from build123d import *

# Parameters (mm, degrees)
SKETCH1_W           = 72
SKETCH1_H           = 39
BOSS_EXTRUDE1_DEPTH = 1.5
SKETCH2_R           = 10
BOSS_EXTRUDE2_DEPTH = 16.8
SKETCH3_R           = 1.6
CUT_EXTRUDE1_DEPTH  = 16.8
SKETCH4_R           = 1.6
CUT_EXTRUDE2_DEPTH  = 16.8
FILLET1_R           = 0.2


with BuildPart() as part:
    # Sketch1 → Boss-Extrude1 (new body)
    with BuildSketch(Plane(origin=(0, 0, 0), x_dir=(1, 0, 0), z_dir=(0, 1, 0))):
        with Locations((36, 19.5)):
            Rectangle(SKETCH1_W, SKETCH1_H)
    extrude(amount=BOSS_EXTRUDE1_DEPTH)

    # Sketch2 → Boss-Extrude2 (add)
    with BuildSketch(Plane(origin=(0, 1.5, 0), x_dir=(1, 0, 0), z_dir=(0, 1, 0))):
        with Locations((36, 19.5)):
            Circle(SKETCH2_R)
    extrude(amount=BOSS_EXTRUDE2_DEPTH)

    # Sketch3 → Cut-Extrude1 (cut)
    with BuildSketch(Plane(origin=(0, 1.5, 0), x_dir=(1, 0, 0), z_dir=(0, 1, 0))):
        with Locations((44, 5.75)):
            Circle(SKETCH3_R)
        with Locations((28, 5.75)):
            Circle(SKETCH3_R)
        with Locations((28, 33.25)):
            Circle(SKETCH3_R)
        with Locations((44, 33.25)):
            Circle(SKETCH3_R)
    extrude(amount=-CUT_EXTRUDE1_DEPTH, mode=Mode.SUBTRACT)

    # Sketch4 → Cut-Extrude2 (cut)
    with BuildSketch(Plane(origin=(0, 1.5, 0), x_dir=(1, 0, 0), z_dir=(0, 1, 0))):
        with Locations((51.75, 3.75)):
            Circle(SKETCH4_R)
        with Locations((51.75, 35.25)):
            Circle(SKETCH4_R)
        with Locations((20.25, 3.75)):
            Circle(SKETCH4_R)
        with Locations((20.25, 35.25)):
            Circle(SKETCH4_R)
    extrude(amount=-CUT_EXTRUDE2_DEPTH, mode=Mode.SUBTRACT)

    # Fillet1
    fillet1_edges = [part.edges().sort_by_distance(p)[0] for p in [
        (26, 18.3, -19.5),
    ]]
    fillet(fillet1_edges, radius=FILLET1_R)


solid = part.part
Could you check a few things on this model? Use its own coordinates, in mm. A direction names the side the tool comes from. Give positions to 0.01 mm unless a question says otherwise; leave off trailing zeros. Loops run counter-clockwise (first coordinate to the right, second up) from the corner with the lowest first, then second, coordinate; pieces in that order, holes last. Notation, with made-up numbers: (44.25, -15.5) -> (81.25, -15.5) arc R24 ccw to (81.25, 23.5) -> close; hole circle Ø1 at (78.25, 63.25). An arc over 180 degrees is marked (long way). Answer as CSV lines item,"result". Start each with the question number.
(1) If we section it at B-B on x = 36: Write out the boundary of the cut face in (y, z), then the cut area to 3 significant figures.
(2) I need wall thicknesses on probe 1 along X at (y, z) = (0.85, -33.25); probe 2 along X at (y, z) = (0.8, -35.25); probe 3 along Z at (x, y) = (20.25, 1.15). Which ranges of each line are inside material? Lowest first, please.
(3) If we section it at A-A on x = 51.75: Write out the boundary of the cut face in (y, z).
(4) If we section it at C-C on y = 16.75: Write out the boundary of the cut face in (x, z), then the cut area to 3 significant figures.
(5) Which directions (+Z, -Z, +X, -X, +Y, -Y) give clear straight access to the entire face, cutting with the end or side of a thin tool? Please do faces 1 (the cylindrical face through (34.698, 9.684, -29.415)), 2 (the cylindrical face through (19.9, 0.76, -33.69)).
(6) I'm going to push flat-ended pins straight in: pin 1 Ø2.5 at (x, z) = (28, -5.75) entering from +Y; pin 2 Ø3.5 at (x, z) = (28, -33.25) entering from +Y; pin 3 Ø2 at (y, z) = (7, -19.5) entering from +X; pin 4 Ø2 at (y, z) = (5, -15.5) entering from +X. Where does each tip first touch, or does it pass through?
(7) If we section it at D-D on x = 28: Count the separate pieces of the cut face and the enclosed holes in it, then the cut area to 3 significant figures.
Computed:
1,outline,"(0, -39) -> (1.5, -39) -> (1.5, -29.5) -> (18.1, -29.5) arc R0.2 ccw to (18.3, -29.3) -> (18.3, -9.7) arc R0.2 ccw to (18.1, -9.5) -> (1.5, -9.5) -> (1.5, 0) -> (0, 0) -> close"
1,area,"394 mm2"
2,probe 1,"x = 0 to 26.4, 29.6 to 42.4, 45.6 to 72"
2,probe 2,"x = 0 to 18.65, 21.85 to 50.15, 53.35 to 72"
2,probe 3,"z = -39 to -36.85, -33.65 to -5.35, -2.15 to 0"
3,outline,"(0, -39) -> (1.5, -39) -> (1.5, -36.85) -> (0, -36.85) -> close; (0, -33.65) -> (1.5, -33.65) -> (1.5, -5.35) -> (0, -5.35) -> close; (0, -2.15) -> (1.5, -2.15) -> (1.5, 0) -> (0, 0) -> close"
4,outline,"circle Ø20 at (36, -19.5)"
4,area,"314 mm2"
5,face 1,"+Y"
5,face 2,"+Y, -Y"
6,pin 1,"passes through"
6,pin 2,"stops at y = 1.5"
6,pin 3,"stops at x = 46"
6,pin 4,"stops at x = 45.54"
7,separate pieces,"3"
7,enclosed holes,"0"
7,area,"250 mm2"
